Check sheet for the modelled part. Datum: model origin and axes. Units: mm. Give positions to 0.01 mm unless a question says otherwise; leave off trailing zeros. Order: outer loops, then holes, each group sorted by start corner. A loop starts at its lowest first (then second) coordinate and runs counter-clockwise, first axis right, second up.
Autodesk Inventor part; units mm, degrees
ref_plane "YZ Plane" through (0, 0, 0) normal (1, 0, 0) x (0, 1, 0)
ref_plane "XZ Plane" through (0, 0, 0) normal (0, 1, 0) x (-1, 0, 0)
ref_plane "XY Plane" through (0, 0, 0) normal (0, 0, 1) x (1, 0, 0)
sketch "Sketch1" plane through (0, 0, 0) normal (0, 0, 1) x (1, 0, 0)
  line L0 (-63.5, -12.7) -> (63.5, -12.7)
  line L1 (63.5, -12.7) -> (63.5, 12.7)
  line L2 (63.5, 12.7) -> (-63.5, 12.7)
  line L3 (-63.5, 12.7) -> (-63.5, -12.7)
  line L4 (-63.5, -12.7) -> (63.5, 12.7) construction
  line L5 (63.5, -12.7) -> (-63.5, 12.7) construction
  point P0 (0, 0)
  dimension "d0" = 127
  dimension "d1" = 25.4
extrude "Extrusion1" add sketch "Sketch1" along normal blind 19.05
sketch "Sketch3" plane through (-63.5, 12.7, 0) normal (0, 1, 0) x (1, 0, 0)
  circle A0 centre (119.38, -9.1052) radius 3.81
  line L0 (0, 0) -> (0, -19.05)
  line L1 (127, 0) -> (127, -19.05)
  point P0 (63.5, 0)
  dimension "d12" = 7.62
  dimension "d14" = 7.62
extrude "Extrusion3" cut sketch "Sketch3" against normal blind 25.4
properties part number "Side Bar"
1) Section check C-C, the plane y = 8.25. Record the cut outline in (x, z).
Recorded:
outline: (-63.5, 0) - (63.5, 0) - (63.5, 19.05) - (-63.5, 19.05) - close; hole circle Ø7.62 at (55.88, 9.11)
2) Draft check along X on faces 1 (the face through (63.5, 0, 9)), 2 (the face through (59.4, 0.18, 10.56)), 3 (the face through (-1, 0, 0)). Enter one of: +X half, -X half, draft (parallel to the pull), parting line (faces both ways), or undercut.
Recorded:
face 1: +X half
face 2: undercut
face 3: draft
3) Section check A-A, the plane x = 55.88. Record the cut outline in (y, z), then the cut area to 3 significant figures.
Recorded:
outline: (-12.7, 0) - (12.7, 0) - (12.7, 5.3) - (-12.7, 5.3) - close; (-12.7, 12.92) - (12.7, 12.92) - (12.7, 19.05) - (-12.7, 19.05) - close
area: 290 mm2
4) Material ranges on L1, parallel to Z at x = 55.88, y = -3.25; L2, parallel to X at y = -10.25, z = 6.75, recorded low to high.
Recorded:
L1: z = 0 to 5.3, 12.92 to 19.05
L2: x = -63.5 to 52.89, 58.87 to 63.5
5) Section check B-B, the plane z = 10.75. Record the cut outline in (x, y), then the cut area to 3 significant figures.
Recorded:
outline: (-63.5, -12.7) - (52.44, -12.7) - (52.44, 12.7) - (-63.5, 12.7) - close; (59.32, -12.7) - (63.5, -12.7) - (63.5, 12.7) - (59.32, 12.7) - close
area: 3,050 mm2
6) Depth check by flat-ended pin: pin 1 Ø6 at (x, z) = (55.88, 9.11) entering from +Y. Enter the tip coordinate at first touch or a pass-through.
Recorded:
pin 1: passes through
